```python
from build123d import *

# Parameters (mm, degrees)
BOSS_EXTRUDE1_DEPTH = 3


with BuildPart() as part:
    # Sketch1 → Boss-Extrude1 (new body)
    with BuildSketch(Plane(origin=(0, 0, 0), x_dir=(1, 0, 0), z_dir=(0, 1, 0))):
        with BuildLine():
            ThreePointArc((34.422746677, -63.95), (40.577345115, -62.107399108), (44.706859879, -57.185878226))
            Line((44.706859879, -57.185878226), (58.490893839, -25.229057412))
            ThreePointArc((58.490893839, -25.229057412), (0, 63.7), (-58.490893839, -25.229057412))
            Line((-58.490893839, -25.229057412), (-44.706859879, -57.185878226))
            ThreePointArc((-44.706859879, -57.185878226), (-40.577345115, -62.107399108), (-34.422746677, -63.95))
            Line((-34.422746677, -63.95), (34.422746677, -63.95))
        make_face()
        with BuildLine():
            Line((34.422746677, -62.75), (-34.422746677, -62.75))
            ThreePointArc((-34.422746677, -62.75), (-39.917923854, -61.104820632), (-43.604990608, -56.710605559))
            Line((-43.604990608, -56.710605559), (-57.389024568, -24.753784745))
            ThreePointArc((-57.389024568, -24.753784745), (-12.637957994, 61.208921063), (62.5, 0))
            ThreePointArc((62.5, 0), (61.208921063, -12.637957994), (57.389024568, -24.753784745))
            Line((57.389024568, -24.753784745), (43.604990608, -56.710605559))
            ThreePointArc((43.604990608, -56.710605559), (39.917923854, -61.104820632), (34.422746677, -62.75))
        make_face(mode=Mode.SUBTRACT)
    extrude(amount=BOSS_EXTRUDE1_DEPTH)


solid = part.part
```
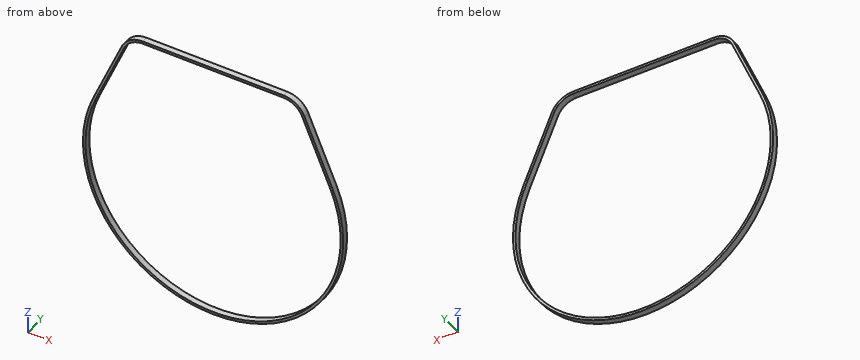
CAD build for the part. Positions are in the model's coordinates, mm. Coordinates: 2 decimals unless noted, no trailing zeros. Order: outer loops, then holes, each group sorted by start corner. A loop starts at its lowest first (then second) coordinate and runs counter-clockwise, first axis right, second up. Notation, with made-up numbers: (84, 30.25) - (137, 30.25) arc R7 cw to (137, 36.25) - close; hole circle Ø10 at (88.5, 32). An arc over 180 degrees is marked (long way). Use a Markdown table: item, result. Add a question column.
(1) Saw through at C-C (y = 0.8). Give the cut face in (x, z) (3 decimals).
(2) Saw through at A-A (z = 18). Give the cut face in (x, y).
(3) Saw through at B-B (x = 0). Give the cut face in (y, z).
(4) Drill centre lines: line 1 along X through (y, z) = (1.35, -1.5); line 2 along Z through (x, y) = (39, 1.55); line 3 along Z through (x, y) = (39.5, 0.4). Where is each one in solid material? Low to high. Write a range as [from, to].
(5) Flat gauge pins, fed straight in: pin 1 (0.9 mm diameter, centred on x = 5, y = 1.5, fed in from -Z); pin 2 (1 mm diameter, centred on x = -43.5, y = 1, fed in from -Z); pin 3 (1.5 mm diameter, centred on y = 2, z = 25, fed in from +X). Where does each tip first touch, or does it go through?
Solved:
| question | item | result |
|---|---|---|
| 1 | outline | (-58.491, 25.229) arc R63.7 ccw (long way) to (58.491, 25.229) - (44.707, 57.186) arc R11.2 ccw to (34.423, 63.95) - (-34.423, 63.95) arc R11.2 ccw to (-44.707, 57.186) - close; hole (-57.389, 24.754) arc R62.5 ccw (long way) to (57.389, 24.754) - (43.605, 56.711) arc R10 ccw to (34.423, 62.75) - (-34.423, 62.75) arc R10 ccw to (-43.605, 56.711) - close |
| 2 | outline | (-61.1, 0) - (-59.85, 0) - (-59.85, 3) - (-61.1, 3) - close; (59.85, 0) - (61.1, 0) - (61.1, 3) - (59.85, 3) - close |
| 3 | outline | (0, -63.7) - (3, -63.7) - (3, -62.5) - (0, -62.5) - close; (0, 62.75) - (3, 62.75) - (3, 63.95) - (0, 63.95) - close |
| 4 | line 1 | x = [-63.68, -62.48], [62.48, 63.68] |
| 4 | line 2 | z = [-50.37, -48.84], [61.64, 62.97] |
| 4 | line 3 | z = [-49.97, -48.44], [61.37, 62.73] |
| 5 | pin 1 | stops at z = -63.54 |
| 5 | pin 2 | stops at z = -47 |
| 5 | pin 3 | stops at x = 58.9 |
